Can you work these out from the drawing? Everything is in mm from the part's minimum corner. Round coordinates to 2 decimals unless told otherwise and drop trailing zeros. Loops run counter-clockwise (first coordinate to the right, second up) from the corner with the lowest first, then second, coordinate; pieces in that order, holes last. Notation, with made-up numbers: (30, 38.5) - (59, 38.5) arc R32 ccw to (59, 64.5) - close; hole circle Ø10 at (17.25, 29.5). An arc over 180 degrees is marked (long way). Answer as a JSON object with one key per item and string values. Group by question number.
1) If we mould it in two halves opening along Y, with no side actions, what happens to the marked faces 1, 2, 3 and 4? For each: pulls with the +Y half, pulls with the -Y half, needs draft (parallel to the pull), parting line crosses it, or undercut.
2) I want a section at C-C, the plane z = 25.5. Please give me the cut outline in (x, y), then the cut area to 3 significant figures.
3) I want a section at D-D, the plane x = 3.5. Please give me the cut outline in (y, z), then the cut area to 3 significant figures.
4) Will these pins go through, and if not, where does the flat tip stop? P1, Ø2, axis at y = 11.5, z = 4, coming from the -X side; P2, Ø1.2, axis at y = 39, z = 5, coming from the -X side (1 decimal); P3, Ø2, axis at x = 13.5, z = 5, coming from the -Y side; P4, Ø3, axis at y = 11.5, z = 20, coming from the -X side.
5) If I drill on line 1 along Z through (x, y) = (19.5, 15); line 2 along Z through (x, y) = (4, 25.5); line 3 along Y through (x, z) = (20.5, 9.5) (1 decimal), over which ranges is the centre line in solid material (lowest first)? Write a range as [from, to].
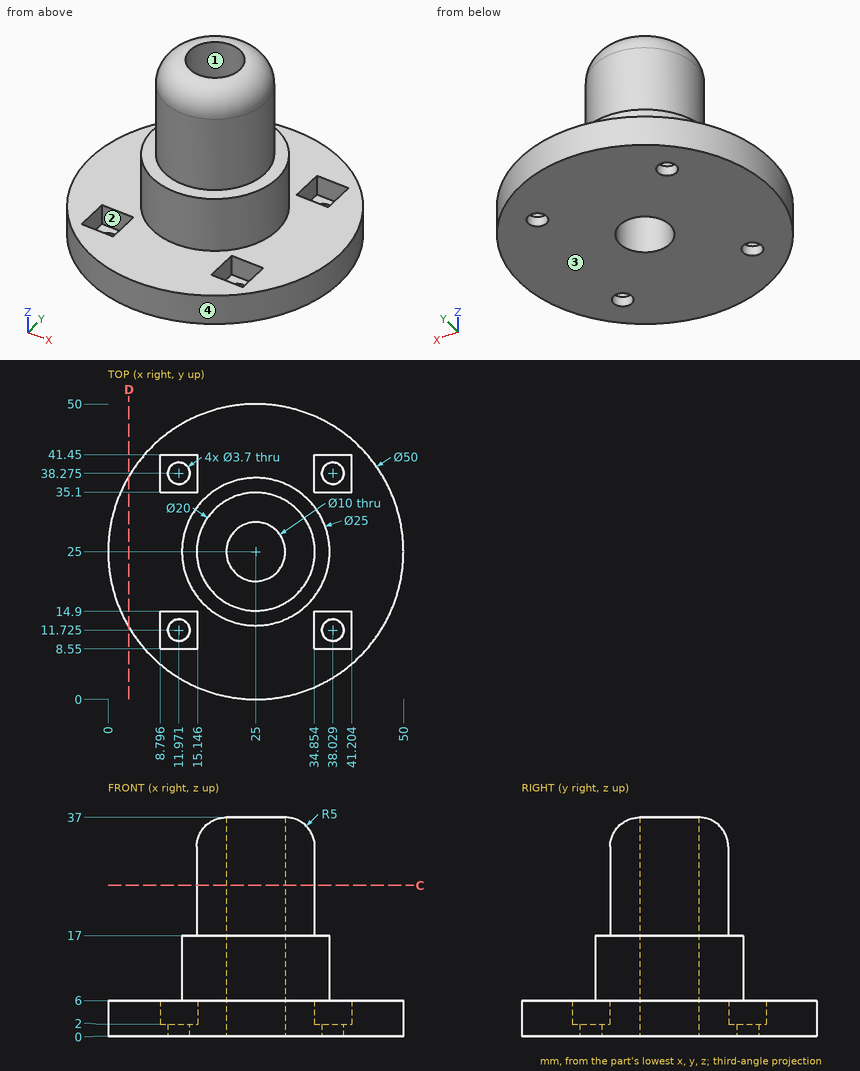
Outcome:
{
 "1": {"face 1": "undercut", "face 2": "undercut", "face 3": "needs draft", "face 4": "parting line crosses it"},
 "2": {"outline": "circle Ø20 at (25, 25); hole circle Ø10 at (25, 25)", "area": "236 mm^2"},
 "3": {"outline": "(12.24, 0) - (37.76, 0) - (37.76, 6) - (12.24, 6) - close", "area": "153 mm^2"},
 "4": {"P1": "x = 3.35", "P2": "x = 3.9", "P3": "y = 2.31", "P4": "through"},
 "5": {"line 1": "[0, 17]", "line 2": "[0, 6]", "line 3": "[13.3, 22.8], [27.2, 36.7]"}
}
